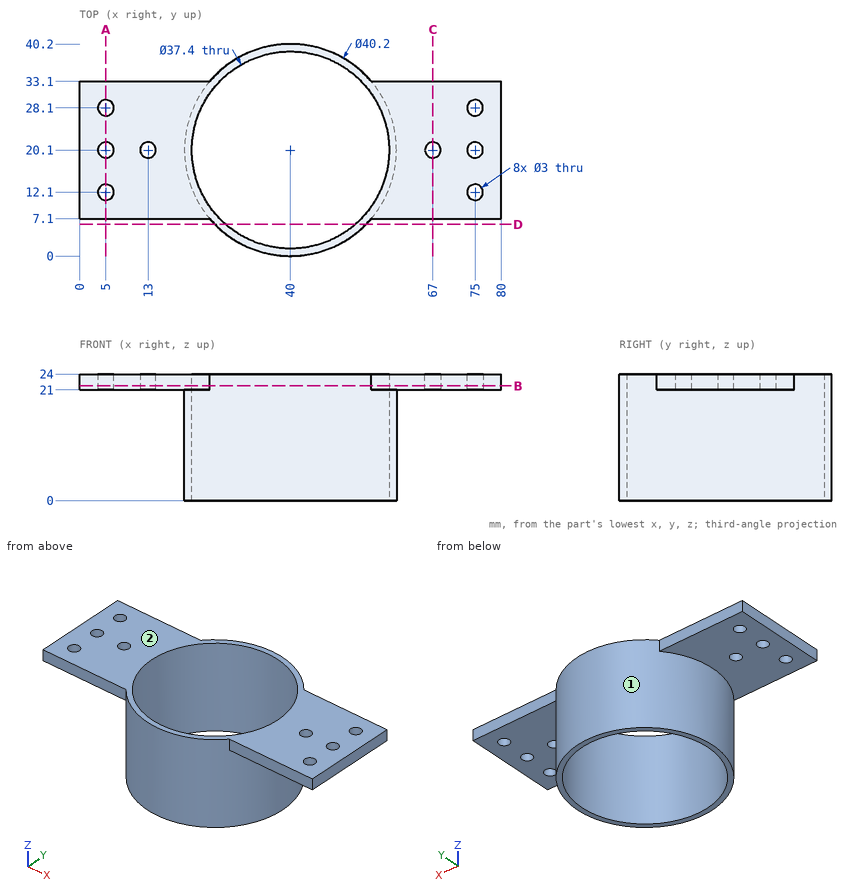
Source: three-view drawing plus pictorial views. Frame: mm from the lowest corner of the part. A direction names the side the tool comes from. Give positions to 0.01 mm unless a question says otherwise; leave off trailing zeros. Order: outer loops, then holes, each group sorted by start corner. A loop starts at its lowest first (then second) coordinate and runs counter-clockwise, first axis right, second up. Notation, with made-up numbers: M 36.5,54.25 L 88.5,54.25 A16 cw 88.5,59.25 Z; hole C 19,-22.5 d1. An arc over 180 degrees is marked long. Return JSON: item names as keys, results as strings.
1) Section query A-A on x = 5. Output: boundary loops of the cut face in (y, z), and give its area (3 significant figures).
Taken from the geometry:
{"outline": "M 7.1,21 L 10.6,21 L 10.6,24 L 7.1,24 Z; M 13.6,21 L 18.6,21 L 18.6,24 L 13.6,24 Z; M 21.6,21 L 26.6,21 L 26.6,24 L 21.6,24 Z; M 29.6,21 L 33.1,21 L 33.1,24 L 29.6,24 Z", "area": "51.0 mm2"}
2) Contact query for flat-ended pins moving along their axis: pin 1 (1.5 mm diameter, centred on x = 12.5, z = 22.5, fed in from +Y); pin 2 (2.5 mm diameter, centred on x = 12, z = 22.5, fed in from -Y); pin 3 (1 mm diameter, centred on x = 24, z = 16, fed in from +Y). Output: stop coordinate, or through.
Taken from the geometry:
{"pin 1": "stops at y = 33.1", "pin 2": "stops at y = 7.1", "pin 3": "stops at y = 32.9"}
3) Section query D-D on y = 6. Output: boundary loops of the cut face in (x, z), and give its area (3 significant figures).
Taken from the geometry:
{"outline": "M 25.68,0 L 27.72,0 L 27.72,24 L 25.68,24 Z; M 52.28,0 L 54.32,0 L 54.32,24 L 52.28,24 Z", "area": "98.0 mm2"}
4) Section query B-B on z = 21.75. Count the separate pieces of the cut face and the enclosed holes in it, and give its area (3 significant figures).
Taken from the geometry:
{"separate pieces": "1", "enclosed holes": "9", "area": "1,230 mm2"}
5) Section query C-C on x = 67. Output: boundary loops of the cut face in (y, z).
Taken from the geometry:
{"outline": "M 7.1,21 L 18.6,21 L 18.6,24 L 7.1,24 Z; M 21.6,21 L 33.1,21 L 33.1,24 L 21.6,24 Z"}
6) Access query for the marked faces 1 and 2. Directions: +Z, -Z, +X, -X, +Y, -Y. A direction counts if a zero-diameter tool reaches every point of the face in a straight line with its end or side. Return the directions, or none.
Taken from the geometry:
{"face 1": "-Z", "face 2": "+Z, +X, -X, +Y, -Y"}
7) Line query: L1, parallel to Y at x = 5, z = 21.8; L2, parallel to Y at x = 40, z = 8.75; L3, parallel to Y at x = 13, z = 22.6. Output: solid intervals per line, ascending. Write a range as [from, to].
Taken from the geometry:
{"L1": "y = [7.1, 10.6], [13.6, 18.6], [21.6, 26.6], [29.6, 33.1]", "L2": "y = [0, 1.4], [38.8, 40.2]", "L3": "y = [7.1, 18.6], [21.6, 33.1]"}
